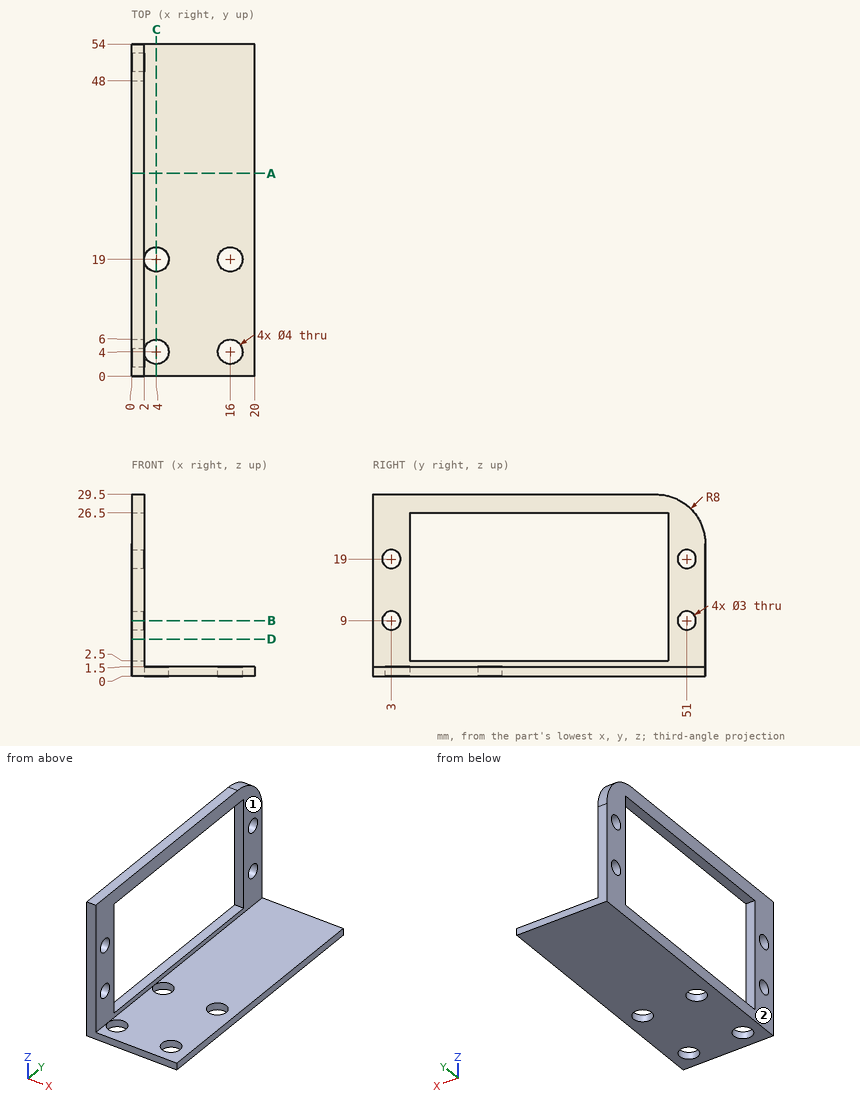
Design review of the part shown in the three views and the two pictorial views. Dimensions are in mm from the part's minimum x, y and z. A direction names the side the tool comes from. Give positions to 0.01 mm unless a question says otherwise; leave off trailing zeros. Write each loop counter-clockwise with the first axis right and the second up, starting at its lowest first coordinate (ties: lowest second). Pieces come first, ordered by that corner, then holes. Notation, with made-up numbers: M 79,17 L 125,17 A20 cw 125,53 Z; hole C 7,12.5 d9. An arc over 180 degrees is marked long. Return JSON: item names as keys, results as strings. Group by question number.
Item 1: Take a section at A-A (y = 33). Give the boundary of the cut face in (x, z), plus the area to 3 significant figures.
Item 2: Wall thickness on line 1 along Y through (x, z) = (1.3, 19); line 2 along Z through (x, y) = (0.7, 3); line 3 along Y through (x, z) = (4, 0.7): over which ranges is each line inside the solid? List them lowest first.
Item 3: Take a section at D-D (z = 6). Give the boundary of the cut face in (x, y).
Item 4: Take a section at B-B (z = 9). Give the boundary of the cut face in (x, y).
Item 5: Take a section at C-C (x = 4). Give the boundary of the cut face in (y, z).
Item 6: Clearance check with flat-ended pins moving along their axes: pin 1 Ø1.8 at (y, z) = (3, 19) entering from -X; pin 2 Ø14 at (y, z) = (16.5, 22) entering from +X; pin 3 Ø4 at (x, y) = (5, 40) entering from +Z. State where each tip first meets the part, or that it passes through.
Item 7: Tool access review of the marked faces 1 and 2: name each direction out of +Z, -Z, +X, -X, +Y, -Y from which nothing blocks a thin tool from reaching the whole face with its end or side.
Return value:
{
 "1": {"outline": "M 0,0 L 20,0 L 20,1.5 L 2,1.5 L 2,2.5 L 0,2.5 Z; M 0,26.5 L 2,26.5 L 2,29.5 L 0,29.5 Z", "area": "38.0 mm2"},
 "2": {"line 1": "y = 0 to 1.5, 4.5 to 6, 48 to 49.5, 52.5 to 54", "line 2": "z = 0 to 7.5, 10.5 to 17.5, 20.5 to 29.5", "line 3": "y = 0 to 2, 6 to 17, 21 to 54"},
 "3": {"outline": "M 0,0 L 2,0 L 2,6 L 0,6 Z; M 0,48 L 2,48 L 2,54 L 0,54 Z"},
 "4": {"outline": "M 0,0 L 2,0 L 2,1.5 L 0,1.5 Z; M 0,4.5 L 2,4.5 L 2,6 L 0,6 Z; M 0,48 L 2,48 L 2,49.5 L 0,49.5 Z; M 0,52.5 L 2,52.5 L 2,54 L 0,54 Z"},
 "5": {"outline": "M 0,0 L 2,0 L 2,1.5 L 0,1.5 Z; M 6,0 L 17,0 L 17,1.5 L 6,1.5 Z; M 21,0 L 54,0 L 54,1.5 L 21,1.5 Z"},
 "6": {"pin 1": "passes through", "pin 2": "stops at x = 2", "pin 3": "stops at z = 1.5"},
 "7": {"face 1": "+Z, +X, +Y, -Y", "face 2": "+Z, -Z, -X, +Y, -Y"}
}
